Geometry check sheet. Reference: the model listing, model coordinates, mm. A direction names the side the tool comes from. Round coordinates to 2 decimals unless told otherwise and drop trailing zeros. Order: outer loops, then holes, each group sorted by start corner. A loop starts at its lowest first (then second) coordinate and runs counter-clockwise, first axis right, second up. Notation, with made-up numbers: (14, -20) - (46, -20) arc R21 ccw to (46, -2) - close; hole circle Ø4 at (67.5, -7.5). An arc over 180 degrees is marked (long way). One line per question, with ' | ' between items. Start each with the question number.
Q1. Gauge pin test, flat ends, axial feed: P1, Ø15, axis at y = -1, z = 36.5, coming from the +X side (3 decimals); P2, Ø10.5, axis at x = 43, y = -2.5, coming from the +Z side. Record the tip position at first contact, or that the pin passes through.
Q2. Sectioned sample at C-C, the plane z = 30.5. Enter the section's corners in (x, y) (1 decimal), then the cut area to 3 significant figures.
Q3. Sectioned sample at B-B, the plane x = 14. Enter the section's corners in (y, z), then the cut area to 3 significant figures.
Q4. Material ranges on line 1 along Z through (x, y) = (1, 11.5); line 2 along X through (y, z) = (-3, 35) (1 decimal), recorded low to high.
Q5. Sectioned sample at A-A, the plane y = 6. Enter the section's corners in (x, z) (1 decimal), then the cut area to 3 significant figures.
Q6. Tool access check on faces 1 (the face through (-60, 0, 53.181)), 2 (the face through (-41.275, 0, 38)). Record the directions out of +Z, -Z, +X, -X, +Y, -Y that give a thin tool (end or side, any length) a straight path to the whole face; none if there is none.
```python
from build123d import *

# Parameters (mm, degrees)
F0_W     = 36.5125
F0_H     = 30.1625
F1_DEPTH = 17.4625


with BuildPart() as f1:
    # F0 (on Front) → F1 (new body, symmetric)
    with BuildSketch(Plane.XZ):
        Polygon((77.7875, -23.01875), (77.7875, 23.01875), (-41.275, 23.01875), (-77.7875, 23.01875), (-77.7875, -23.01875), align=None)
        with Locations((-59.53125, 38.1)):
            Rectangle(F0_W, F0_H)
    extrude(amount=F1_DEPTH, both=True)


solid = f1.part
```
Determined:
1) P1: stops at x = -41.275 | P2: stops at z = 23.02
2) outline: (-77.8, -17.5) - (-41.3, -17.5) - (-41.3, 17.5) - (-77.8, 17.5) - close | area: 1,280 mm2
3) outline: (-17.46, -23.02) - (17.46, -23.02) - (17.46, 23.02) - (-17.46, 23.02) - close | area: 1,610 mm2
4) line 1: z = -23.02 to 23.02 | line 2: x = -77.8 to -41.3
5) outline: (-77.8, -23) - (77.8, -23) - (77.8, 23) - (-41.3, 23) - (-41.3, 53.2) - (-77.8, 53.2) - close | area: 8,260 mm2
6) face 1: +Z, +X, -X, +Y, -Y | face 2: +Z, +X, +Y, -Y
